from build123d import *

# Parameters (mm, degrees)
IZIM1_R                     = 5
IZIM1_R_2                   = 2.5
Y_KSEKLIK_EKSTR_ZYON2_DEPTH = 1
IZIM2_R                     = 3
Y_KSEKLIK_EKSTR_ZYON4_DEPTH = 1


with BuildPart() as part:
    # Çizim1 → Yükseklik-Ekstrüzyon2 (new body)
    with BuildSketch(Plane.XY):
        with BuildLine():
            Line((-25, 43.301270189), (-26.146521576, 40.39207739))
            ThreePointArc((-26.146521576, 40.39207739), (-27.544598222, 38.602623821), (-29.691484877, 37.862596744))
            Line((-29.691484877, 37.862596744), (-32.693673826, 37.730024144))
            Line((-32.693673826, 37.730024144), (-33.252115355, 34.777253066))
            ThreePointArc((-33.252115355, 34.777253066), (-34.290118058, 32.757522199), (-36.260310201, 31.628316593))
            Line((-36.260310201, 31.628316593), (-39.184480502, 30.935538106))
            Line((-39.184480502, 30.935538106), (-39.17973637, 27.930427214))
            ThreePointArc((-39.17973637, 27.930427214), (-39.820893366, 25.751969023), (-41.54459596, 24.273587558))
            Line((-41.54459596, 24.273587558), (-44.287157421, 23.045145208))
            Line((-44.287157421, 23.045145208), (-43.719395692, 20.094152054))
            ThreePointArc((-43.719395692, 20.094152054), (-43.940993675, 17.834139505), (-45.357143694, 16.058954583))
            Line((-45.357143694, 16.058954583), (-47.82093971, 14.338366552))
            Line((-47.82093971, 14.338366552), (-46.710273625, 11.546031539))
            ThreePointArc((-46.710273625, 11.546031539), (-46.504462376, 9.284526705), (-47.562892001, 7.275425136))
            Line((-47.562892001, 7.275425136), (-49.660641368, 5.123644113))
            Line((-49.660641368, 5.123644113), (-48.046416828, 2.588887101))
            ThreePointArc((-48.046416828, 2.588887101), (-47.420487313, 0.406004917), (-48.083701146, -1.765839874))
            Line((-48.083701146, -1.765839874), (-49.741090048, -4.272585973))
            Line((-49.741090048, -4.272585973), (-47.680491761, -6.459969953))
            ThreePointArc((-47.680491761, -6.459969953), (-46.656617846, -8.486899797), (-46.901121207, -10.744549126))
            Line((-46.901121207, -10.744549126), (-48.059435816, -13.517457571))
            Line((-48.059435816, -13.517457571), (-45.625461503, -15.279979352))
            ThreePointArc((-45.625461503, -15.279979352), (-44.239914432, -17.079151855), (-44.057045667, -19.342627369))
            Line((-44.057045667, -19.342627369), (-44.675252109, -22.283466496))
            Line((-44.675252109, -22.283466496), (-41.954126526, -23.558687864))
            ThreePointArc((-41.954126526, -23.558687864), (-40.255989993, -25.066366444), (-39.652227319, -27.255483394))
            Line((-39.652227319, -27.255483394), (-39.708425324, -30.260072511))
            Line((-39.708425324, -30.260072511), (-36.7965457, -31.002818113))
            ThreePointArc((-36.7965457, -31.002818113), (-34.84597704, -32.165592505), (-33.842709051, -34.202800331))
            Line((-33.842709051, -34.202800331), (-33.334907776, -37.164700371))
            Line((-33.334907776, -37.164700371), (-30.335428898, -37.348658075))
            ThreePointArc((-30.335428898, -37.348658075), (-28.201527977, -38.125336415), (-26.834295942, -39.938466016))
            Line((-26.834295942, -39.938466016), (-25.73775467, -42.866863479))
            ThreePointArc((-25.73775467, -42.866863479), (-24.554196145, -43.55561332), (-23.352220135, -44.21169319))
            ThreePointArc((-23.352220135, -44.21169319), (-17.219408632, -49.939828574), (-14.829333353, -57.984109281))
            ThreePointArc((-14.829333353, -57.984109281), (-20.099106379, -76.543069457), (-25, -57.883306535))
            Line((-25, -57.883306535), (-25, -57.052607302))
            ThreePointArc((-25, -57.052607302), (-25.590454576, -54.960957236), (-27.1875, -53.486819346))
            ThreePointArc((-27.1875, -53.486819346), (-59.999999835, 0.004450967), (-27.179564099, 53.490852446))
            ThreePointArc((-27.179564099, 53.490852446), (-24.232021318, 53.76021953), (-21.906244367, 51.929556087))
            ThreePointArc((-21.906244367, 51.929556087), (-21.212806241, 47.755648425), (-23.446136356, 44.161959762))
            ThreePointArc((-23.446136356, 44.161959762), (-24.226890609, 43.73851588), (-25, 43.301270189))
        make_face()
        with Locations((-20, -66.543560573)):
            Circle(IZIM1_R, mode=Mode.SUBTRACT)
        with Locations((-31.620079453, -45.001895242)):
            Circle(IZIM1_R_2, mode=Mode.SUBTRACT)
        with Locations((-55, 0)):
            Circle(IZIM1_R_2, mode=Mode.SUBTRACT)
        with Locations((-28.000624989, 47.338831842)):
            Circle(IZIM1_R_2, mode=Mode.SUBTRACT)
    extrude(amount=Y_KSEKLIK_EKSTR_ZYON2_DEPTH)

    # Çizim2 → Yükseklik-Ekstrüzyon4 (add)
    with BuildSketch(Plane.XY.offset(1)):
        with BuildLine():
            Line((-8, -68.275611381), (-10.601540351, -69.777611403))
            ThreePointArc((-10.601540351, -69.777611403), (-11.025419883, -70.260953374), (-11.067466177, -70.902455852))
            Line((-11.067466177, -70.902455852), (-10.289973754, -73.804097076))
            ThreePointArc((-10.289973754, -73.804097076), (-10.807611845, -75.735948729), (-12.739463497, -76.253586819))
            Line((-12.739463497, -76.253586819), (-15.641104722, -75.476094396))
            ThreePointArc((-15.641104722, -75.476094396), (-16.282607199, -75.51814069), (-16.765949171, -75.942020222))
            Line((-16.765949171, -75.942020222), (-18.267949192, -78.543560573))
            ThreePointArc((-18.267949192, -78.543560573), (-20, -79.543560573), (-21.732050808, -78.543560573))
            Line((-21.732050808, -78.543560573), (-23.234050829, -75.942020222))
            ThreePointArc((-23.234050829, -75.942020222), (-23.717392801, -75.51814069), (-24.358895278, -75.476094396))
            Line((-24.358895278, -75.476094396), (-27.260536503, -76.253586819))
            ThreePointArc((-27.260536503, -76.253586819), (-29.192388155, -75.735948729), (-29.710026246, -73.804097076))
            Line((-29.710026246, -73.804097076), (-28.932533823, -70.902455852))
            ThreePointArc((-28.932533823, -70.902455852), (-28.974580117, -70.260953374), (-29.398459649, -69.777611403))
            Line((-29.398459649, -69.777611403), (-32, -68.275611381))
            ThreePointArc((-32, -68.275611381), (-33, -66.543560573), (-32, -64.811509766))
            Line((-32, -64.811509766), (-29.398459649, -63.309509744))
            ThreePointArc((-29.398459649, -63.309509744), (-28.974580117, -62.826167772), (-28.932533823, -62.184665295))
            Line((-28.932533823, -62.184665295), (-29.710026246, -59.28302407))
            ThreePointArc((-29.710026246, -59.28302407), (-29.192388155, -57.351172418), (-27.260536503, -56.833534328))
            Line((-27.260536503, -56.833534328), (-24.358895278, -57.61102675))
            ThreePointArc((-24.358895278, -57.61102675), (-23.717392801, -57.568980457), (-23.234050829, -57.145100924))
            Line((-23.234050829, -57.145100924), (-21.732050808, -54.543560573))
            ThreePointArc((-21.732050808, -54.543560573), (-20, -53.543560573), (-18.267949192, -54.543560573))
            Line((-18.267949192, -54.543560573), (-16.765949171, -57.145100924))
            ThreePointArc((-16.765949171, -57.145100924), (-16.282607199, -57.568980457), (-15.641104722, -57.61102675))
            Line((-15.641104722, -57.61102675), (-12.739463497, -56.833534328))
            ThreePointArc((-12.739463497, -56.833534328), (-10.807611845, -57.351172418), (-10.289973754, -59.28302407))
            Line((-10.289973754, -59.28302407), (-11.067466177, -62.184665295))
            ThreePointArc((-11.067466177, -62.184665295), (-11.025419883, -62.826167772), (-10.601540351, -63.309509744))
            Line((-10.601540351, -63.309509744), (-8, -64.811509766))
            ThreePointArc((-8, -64.811509766), (-7, -66.543560573), (-8, -68.275611381))
        make_face()
        with Locations((-20, -66.543560573)):
            Circle(IZIM2_R, mode=Mode.SUBTRACT)
    extrude(amount=-Y_KSEKLIK_EKSTR_ZYON4_DEPTH)


solid = part.part
The listing builds one solid part. Answer for the finished solid, in the listing's coordinates (mm). A direction names the side the tool comes from. Give positions to 0.01 mm unless a question says otherwise; leave off trailing zeros. Write each loop counter-clockwise with the first axis right and the second up, starting at its lowest first coordinate (ties: lowest second). Pieces come first, ordered by that corner, then holes.
Item 1: Which of the six approach directions +Z, -Z, +X, -X, +Y, -Y give full straight-line access (tool end or side, diameter ignored) to faces 1 (the cylindrical face through (-28.228, -38.106, 0.493)), 2 (the cylindrical face through (-32.162, -47.442, 0.493))?
Item 2: Section D-D, the plane y = 36 is taken. Write down the section's boundary in (x, z).
Item 3: A flat-ended cylindrical pin translates along its axis: P1, Ø4.5, axis at x = -31.62, y = -45, coming from the -Z side. Find the tip coordinate at first contact, or state that the pin passes through.
Item 4: Find the intervals of material crossed by line 1 along Y through (x, z) = (-20, 0.7); line 2 along Y through (x, z) = (-49, 0.5); line 3 along Y through (x, z) = (-22.5, 0.95), in increasing order.
Item 5: Determine the mould class of faces 3 (the flat face through (-45, -17, 1)), 4 (the cylindrical face through (-39.803, 25.779, 0.493)) for opening direction Y: released by +Y, released by -Y, zero draft, split by the parting line, or undercut.
Item 6: Section A-A, the plane x = -55 is taken. Write down the section's boundary in (y, z), plus the area to 3 significant figures.
Item 7: Section C-C, the plane z = 0.85 is taken. Count the separate pieces of the cut face and the enclosed holes in it, plus the area to 3 significant figures.
Item 8: Section B-B, the plane y = 0 is taken. Write down the section's boundary in (x, z), plus the area to 3 significant figures.
Completed:
1. face 1: +Z, -Z, +X
1. face 2: +Z, -Z
2. outline: (-48, 0) - (-33.02, 0) - (-33.02, 1) - (-48, 1) - close
3. P1: passes through
4. line 1: y = -79.54 to -69.54, -63.54 to -46.58
4. line 2: y = -34.63 to -5.06, -3.15 to 4.09, 5.8 to 34.63
4. line 3: y = -77.21 to -68.2, -64.89 to -44.7, 45.07 to 52.71
5. face 3: zero draft
5. face 4: undercut
6. outline: (-23.98, 0) - (-2.5, 0) - (-2.5, 1) - (-23.98, 1) - close; (2.5, 0) - (23.98, 0) - (23.98, 1) - (2.5, 1) - close
6. area: 43.0 mm2
7. separate pieces: 1
7. enclosed holes: 4
7. area: 1,820 mm2
8. outline: (-60, 0) - (-57.5, 0) - (-57.5, 1) - (-60, 1) - close; (-52.5, 0) - (-47.44, 0) - (-47.44, 1) - (-52.5, 1) - close
8. area: 7.56 mm2
